Geometry check sheet. Reference: drawing and pictorial views, mm from the part's lowest x, y, z. A direction names the side the tool comes from. Give positions to 0.01 mm unless a question says otherwise; leave off trailing zeros. Write each loop counter-clockwise with the first axis right and the second up, starting at its lowest first coordinate (ties: lowest second). Pieces come first, ordered by that corner, then holes. Notation, with made-up numbers: M 12,-33 L 34,-33 A23 ccw 34,-24 Z; hole C 15,-2.75 d11. An arc over 180 degrees is marked long. Write item = value, one per line. Start each with the question number.
1) Access from +Z, -Z, +X, -X, +Y, -Y to the whole of each face (thin tool, end or side, straight path). Record for the marked faces 1 and 2.
2) Scan lines: line 1 along X through (y, z) = (1.6, 1); line 2 along X through (y, z) = (1.8, 1.8); line 3 along Z through (x, y) = (1, 1.35). Record each from-to range of solid material in increasing order. Write a range as [from, to].
3) Cross-section at A-A, the plane x = 1.75. Record the cut outline in (y, z).
4) Go/stop test with flat-tipped pins: pin 1 (0.6 mm diameter, centred on y = 2, z = 1, fed in from -X); pin 2 (2 mm diameter, centred on x = 5.5, z = 3.5, fed in from -Y) (1 decimal). Record where each tip stops, or that it passes through.
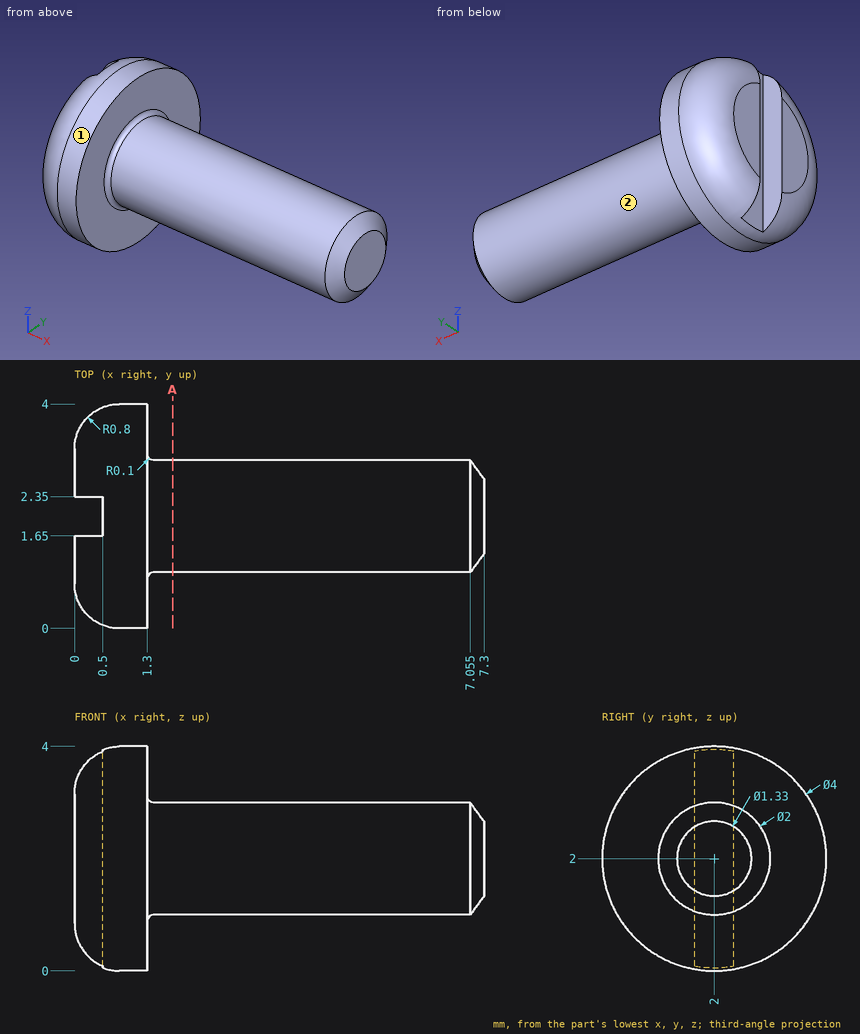
Reply:
q1.face_1 = +X, -X
q1.face_2 = +X
q2.line_1 = [0, 1.3]
q2.line_2 = [0.5, 7.3]
q2.line_3 = [0.11, 3.89]
q3.outline = C 2,2 d2
q4.pin_1 = 0.5
q4.pin_2 = 1.1
